```python
from build123d import *

# Parameters (mm, degrees)
BOSS_EXTRUDE1_DEPTH = 101.6
CUT_EXTRUDE1_START  = -41.3258
SKETCH3_R           = 3.175
SKETCH3_R_2         = 2.921
CUT_EXTRUDE1_DEPTH  = 0.7874
CUT_EXTRUDE2_START  = -28.5496
SKETCH3_3_R         = 3.175
SKETCH3_3_R_2       = 2.921
CUT_EXTRUDE2_DEPTH  = 0.7874
CUT_EXTRUDE3_START  = -11.8872
SKETCH3_4_R         = 3.175
SKETCH3_4_R_2       = 2.921
CUT_EXTRUDE3_DEPTH  = 0.7874


with BuildPart() as part:
    # Sketch1 → Boss-Extrude1 (new body)
    with BuildSketch(Plane(origin=(0, 0, 0), x_dir=(1, 0, 0), z_dir=(0, 1, 0))):
        with BuildLine():
            Line((-1.190625, 2.943303775), (-1.190625, 1.752678775))
            Line((-1.190625, 1.752678775), (1.190625, 1.752678775))
            Line((1.190625, 1.752678775), (1.190625, 2.943303775))
            ThreePointArc((1.190625, 2.943303775), (0, -3.175), (-1.190625, 2.943303775))
        make_face()
    extrude(amount=BOSS_EXTRUDE1_DEPTH)

    # Sketch3 → Cut-Extrude1 (cut)
    with BuildSketch(Plane(origin=(0, 101.6, 0), x_dir=(1, 0, 0), z_dir=(0, 1, 0)).offset(CUT_EXTRUDE1_START)):
        Circle(SKETCH3_R)
        Circle(SKETCH3_R_2, mode=Mode.SUBTRACT)
    extrude(amount=CUT_EXTRUDE1_DEPTH, mode=Mode.SUBTRACT)

    # Sketch3<3> → Cut-Extrude2 (cut)
    with BuildSketch(Plane(origin=(0, 101.6, 0), x_dir=(1, 0, 0), z_dir=(0, 1, 0)).offset(CUT_EXTRUDE2_START)):
        Circle(SKETCH3_3_R)
        Circle(SKETCH3_3_R_2, mode=Mode.SUBTRACT)
    extrude(amount=CUT_EXTRUDE2_DEPTH, mode=Mode.SUBTRACT)

    # Sketch3<4> → Cut-Extrude3 (cut)
    with BuildSketch(Plane(origin=(0, 101.6, 0), x_dir=(1, 0, 0), z_dir=(0, 1, 0)).offset(CUT_EXTRUDE3_START)):
        Circle(SKETCH3_4_R)
        Circle(SKETCH3_4_R_2, mode=Mode.SUBTRACT)
    extrude(amount=CUT_EXTRUDE3_DEPTH, mode=Mode.SUBTRACT)


solid = part.part
```
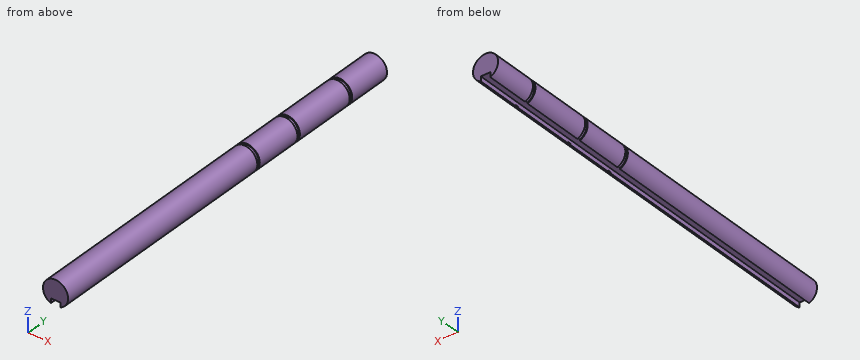
CAD build for the part. Positions are in the model's coordinates, mm. Coordinates: 2 decimals unless noted, no trailing zeros. Write each loop counter-clockwise with the first axis right and the second up, starting at its lowest first coordinate (ties: lowest second). Pieces come first, ordered by that corner, then holes. Notation, with made-up numbers: (6, 54) -> (51, 54) arc R7 cw to (51, 62) -> close; hole circle Ø8 at (78, 79). An arc over 180 degrees is marked (long way). Return JSON: item names as keys, results as strings. Group by question number.
Q1. Cut at A-A, the plane x = 0. Give the cut face in (y, z) (3 decimals).
Q2. Drill centre lines: line 1 (Y direction, x = 0.75, z = 3); line 2 (X direction, y = 91, z = -2); line 3 (X direction, y = 71.5, z = -1.25). Where is each one in solid material? Low to high.
Q3. Flat gauge pins, fed straight in: pin 1 (1 mm diameter, centred on y = 61.5, z = -2.5, fed in from -X); pin 2 (0.7 mm diameter, centred on x = 0.5, y = 39, fed in from -Z); pin 3 (1 mm diameter, centred on y = 76, z = -2, fed in from +X). Where does each tip first touch, or does it go through?
Q4. Cut at B-B, the plane y = 38. Give the cut face in (x, z) (3 decimals).
Q5. Cut at C-C, the plane z = -0.75. Give the cut face in (x, y).
Returned:
{
 "1": {"outline": "(0, -1.753) -> (101.6, -1.753) -> (101.6, 3.175) -> (90.5, 3.175) -> (90.5, 2.921) -> (89.713, 2.921) -> (89.713, 3.175) -> (73.838, 3.175) -> (73.838, 2.921) -> (73.05, 2.921) -> (73.05, 3.175) -> (61.062, 3.175) -> (61.062, 2.921) -> (60.274, 2.921) -> (60.274, 3.175) -> (0, 3.175) -> close"},
 "2": {"line 1": "y = 0 to 60.27, 61.06 to 73.05, 73.84 to 89.71, 90.5 to 101.6", "line 2": "x = -2.47 to -1.19, 1.19 to 2.47", "line 3": "x = -2.92 to 2.92"},
 "3": {"pin 1": "stops at x = -2.47", "pin 2": "stops at z = -1.75", "pin 3": "stops at x = 2.8"},
 "4": {"outline": "(-1.191, -2.943) -> (-1.191, -1.753) -> (1.191, -1.753) -> (1.191, -2.943) arc R3.175 ccw (long way) to start"},
 "5": {"outline": "(-3.09, 0) -> (3.09, 0) -> (3.09, 60.27) -> (2.82, 60.27) -> (2.82, 61.06) -> (3.09, 61.06) -> (3.09, 73.05) -> (2.82, 73.05) -> (2.82, 73.84) -> (3.09, 73.84) -> (3.09, 89.71) -> (2.82, 89.71) -> (2.82, 90.5) -> (3.09, 90.5) -> (3.09, 101.6) -> (-3.09, 101.6) -> (-3.09, 90.5) -> (-2.82, 90.5) -> (-2.82, 89.71) -> (-3.09, 89.71) -> (-3.09, 73.84) -> (-2.82, 73.84) -> (-2.82, 73.05) -> (-3.09, 73.05) -> (-3.09, 61.06) -> (-2.82, 61.06) -> (-2.82, 60.27) -> (-3.09, 60.27) -> close"}
}
